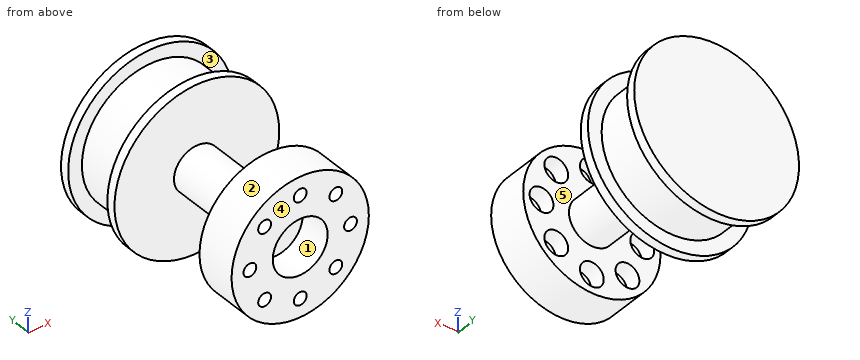
Autodesk Inventor part; units mm, degrees
ref_plane "YZ Plane" through (0, 0, 0) normal (1, 0, 0) x (0, 1, 0)
ref_plane "XZ Plane" through (0, 0, 0) normal (0, 1, 0) x (-1, 0, 0)
ref_plane "XY Plane" through (0, 0, 0) normal (0, 0, 1) x (1, 0, 0)
sketch "Sketch1" plane through (0, 0, 0) normal (0, 1, 0) x (-1, 0, 0)
  circle A0 centre (0, 0) radius 15
  dimension "d0" = 30
extrude "Extrusion1" add sketch "Sketch1" along normal blind 9
sketch "Sketch3" plane through (0, 9, 0) normal (0, 1, 0) x (1, 0, 0)
  circle A0 centre (0, 0) radius 11 construction
  line L0 (0, 0) -> (0, 11) construction
  line L1 (0, 11) -> (7.7782, 7.7782) construction
  line L2 (7.7782, 7.7782) -> (11, 0) construction
  line L3 (11, 0) -> (7.7782, -7.7782) construction
  line L4 (7.7782, -7.7782) -> (0, -11) construction
  line L5 (0, -11) -> (-7.7782, -7.7782) construction
  line L6 (-7.7782, -7.7782) -> (-11, 0) construction
  line L7 (-11, 0) -> (-7.7782, 7.7782) construction
  line L8 (-7.7782, 7.7782) -> (0, 11) construction
  circle A1 centre (-11, 0) radius 1.4
  circle A2 centre (-7.7782, 7.7782) radius 1.4
  circle A3 centre (-7.7782, -7.7782) radius 1.4
  circle A4 centre (0, -11) radius 1.4
  circle A5 centre (7.7782, -7.7782) radius 1.4
  circle A6 centre (11, 0) radius 1.4
  circle A7 centre (7.7782, 7.7782) radius 1.4
  circle A8 centre (0, 11) radius 1.4
  dimension "d12" = 22
  dimension "d13" = 2.8
  dimension "d14" = 2.8
  dimension "d15" = 2.8
  dimension "d16" = 2.8
  dimension "d17" = 2.8
  dimension "d18" = 2.8
  dimension "d19" = 2.8
  dimension "d20" = 2.8
extrude "Extrusion3" cut sketch "Sketch3" against normal up to next
sketch "Sketch4" plane through (0, 9, 0) normal (0, 1, 0) x (1, 0, 0)
  circle A0 centre (-11, 0) radius 1.4 construction
  circle A1 centre (0, 0) radius 11 construction
  line L0 (0, 0) -> (-11, 0) construction
  line L1 (-11, 0) -> (-7.7782, 7.7782) construction
  line L2 (-7.7782, 7.7782) -> (0, 11) construction
  line L3 (0, 11) -> (7.7782, 7.7782) construction
  line L4 (7.7782, 7.7782) -> (11, 0) construction
  line L5 (11, 0) -> (7.7782, -7.7782) construction
  line L6 (7.7782, -7.7782) -> (0, -11) construction
  line L7 (0, -11) -> (-7.7782, -7.7782) construction
  line L8 (-7.7782, -7.7782) -> (-11, 0) construction
  circle A2 centre (-11, 0) radius 2.6
  circle A3 centre (-7.7782, 7.7782) radius 1.4
  circle A4 centre (-7.7782, 7.7782) radius 2.6
  circle A5 centre (0, 11) radius 2.6
  circle A6 centre (7.7782, 7.7782) radius 2.6
  circle A7 centre (11, 0) radius 2.6
  circle A8 centre (7.7782, -7.7782) radius 1.4
  circle A9 centre (7.7782, -7.7782) radius 2.6
  circle A10 centre (0, -11) radius 1.4
  circle A11 centre (0, -11) radius 2.6
  circle A12 centre (-7.7782, -7.7782) radius 2.6
  dimension "d23" = 5.2
  dimension "d24" = 5.2
  dimension "d25" = 5.2
  dimension "d26" = 5.2
  dimension "d27" = 5.2
  dimension "d28" = 5.2
  dimension "d29" = 5.2
  dimension "d30" = 5.2
extrude "Extrusion4" cut sketch "Sketch4" against normal blind 3.5
sketch "Sketch5" plane through (0, 0, 0) normal (0, -1, 0) x (1, 0, 0)
  circle A0 centre (0, 0) radius 6
  dimension "d33" = 12
extrude "Extrusion5" cut sketch "Sketch5" against normal blind 7
sketch "Skizze6" plane through (0, 9, 0) normal (0, 1, 0) x (1, 0, 0)
  circle A0 centre (0, 0) radius 6
  circle A1 centre (0, 0) radius 5
  dimension "d36" = 10
extrude "Extrusion6" add sketch "Skizze6" along normal blind 20 contours A1
sketch "Skizze9" plane through (0, 29, 0) normal (0, 1, 0) x (1, 0, 0)
  circle A0 centre (0, 0) radius 15 construction
  circle A1 centre (0, 0) radius 6 construction
  line L0 (0, 0) -> (0, -15) construction
  line L1 (0, 0) -> (0, -15) construction
  circle A2 centre (0, 0) radius 15
extrude "Extrusion7" add sketch "Skizze9" along normal blind 15
sketch "Skizze10" plane through (0, 44, 0) normal (0, 1, 0) x (1, 0, 0)
  line L0 (0, 0) -> (0, -18) construction
  circle A0 centre (0, 0) radius 5
  circle A1 centre (0, 0) radius 18
  dimension "d44" = 18
extrude "Extrusion8" add sketch "Skizze10" against normal blind 2
ref_plane "Arbeitsebene2" through (0, 36.5, 0) normal (0, 1, 0) x (1, 0, 0)
mirror "Spiegeln1" about plane through (0, 36.5, 0) normal (0, 1, 0) of "Extrusion8"
properties part number "spinning_wheel"
Could you check a few things on this model? Use its own coordinates, in mm. Face numbers are marked on the shaded views. A direction names the side the tool comes from. Give positions to 0.01 mm unless a question says otherwise; leave off trailing zeros. Loops run counter-clockwise (first coordinate to the right, second up) from the corner with the lowest first, then second, coordinate; pieces in that order, holes last. Notation, with made-up numbers: (-6, 42) -> (41, 42) arc R5 cw to (41, 47) -> close; hole circle Ø9 at (-33.75, 29). An arc over 180 degrees is marked (long way). Put each result on its own line as item: value.
(1) I'm going to push flat-ended pins straight in: pin 1 Ø3.5 at (x, z) = (0.5, -1) entering from -Y; pin 2 Ø4 at (y, z) = (37.5, -13.5) entering from -X; pin 3 Ø6 at (y, z) = (14, 0.5) entering from +X. Where does each tip first touch, or does it pass through?
Computed:
pin 1: y = 7
pin 2: x = -9.63
pin 3: x = 5
(2) Imagine slicing it at B-B on z = 11. Write out the boundary of the cut face in (x, y).
Computed:
outline: (-14.25, 29) -> (14.25, 29) -> (14.25, 31) -> (10.2, 31) -> (10.2, 42) -> (14.25, 42) -> (14.25, 44) -> (-14.25, 44) -> (-14.25, 42) -> (-10.2, 42) -> (-10.2, 31) -> (-14.25, 31) -> close; (-10.2, 0) -> (-1.4, 0) -> (-1.4, 5.5) -> (-2.6, 5.5) -> (-2.6, 9) -> (-10.2, 9) -> close; (1.4, 0) -> (10.2, 0) -> (10.2, 9) -> (2.6, 9) -> (2.6, 5.5) -> (1.4, 5.5) -> close
(3) For the marked faces 4 and 5, which set-ups out of +Z, -Z, +X, -X, +Y, -Y let a thin tool reach every point of the face, with its end or its side?
Computed:
face 4: +Z, -Z, +X, -X, -Y
face 5: none
(4) Imagine slicing it at C-C on y = 12. Write out the boundary of the cut face in (x, z), plus the area to 3 significant figures.
Computed:
outline: circle Ø10 at (0, 0)
area: 78.5 mm^2
(5) Please list where these lines run through material, in increasing order: probe 1 along Z at (x, y) = (0, 1); probe 2 along Y at (x, z) = (14.5, 2.5); probe 3 along Y at (x, z) = (-9.5, 15). Write a range as [from, to].
Computed:
probe 1: [-15, -12.4], [-9.6, -6], [6, 9.6], [12.4, 15]
probe 2: [0, 9], [29, 44]
probe 3: [29, 31], [42, 44]
(6) Imagine slicing it at D-D on z = 0. State how many separate pieces and enclosed holes the cut face has, plus the area to 3 significant figures.
Computed:
separate pieces: 3
enclosed holes: 0
area: 793 mm^2
(7) Imagine slicing it at A-A on x = 11. Write out the boundary of the cut face in (y, z), plus the area to 3 significant figures.
Computed:
outline: (0, -10.2) -> (9, -10.2) -> (9, -2.6) -> (5.5, -2.6) -> (5.5, -1.4) -> (0, -1.4) -> close; (0, 1.4) -> (5.5, 1.4) -> (5.5, 2.6) -> (9, 2.6) -> (9, 10.2) -> (0, 10.2) -> close; (29, -14.25) -> (31, -14.25) -> (31, -10.2) -> (42, -10.2) -> (42, -14.25) -> (44, -14.25) -> (44, 14.25) -> (42, 14.25) -> (42, 10.2) -> (31, 10.2) -> (31, 14.25) -> (29, 14.25) -> close
area: 488 mm^2
(8) Thinking about a two-plate mould opening in Z: for the marked faces 1, 2 and 3, which applies, pulls with the +Z half, pulls with the -Z half, needs draft (parallel to the pull), parting line crosses it, or undercut?
Computed:
face 1: undercut
face 2: parting line crosses it
face 3: needs draft
